Source: CAD feature listing. Evaluate the final solid. Frame: model axes, mm. Face numbers are marked on the shaded views. Round coordinates to 2 decimals unless told otherwise and drop trailing zeros. Order: outer loops, then holes, each group sorted by start corner. A loop starts at its lowest first (then second) coordinate and runs counter-clockwise, first axis right, second up. Notation, with made-up numbers: (-5.75, -28) - (35.25, -28) arc R11 ccw to (35.25, -9) - close; hole circle Ø7 at (52, -7.5). An arc over 180 degrees is marked (long way). Use one line per item in the form item = value. Start each with the question number.
Q1. Pin query (flat end, axial travel): pin 1 Ø1.5 at (x, y) = (7.5, 0) entering from +Z; pin 2 Ø1.6 at (x, y) = (-4, 0) entering from -Z; pin 3 Ø2.5 at (x, y) = (1, 0.5) entering from -Z. Return the tip coordinate at first contact, or that it passes through.
Q2. Ray query, line 1 (Y direction, x = -0.25, z = 2.5); line 2 (Z direction, x = -7.75, y = 0.75); line 3 (X direction, y = -1.25, z = 2.5). Return the intervals inside material, ascending. Write a range as [from, to].
Q3. Draft query along Y for the marked faces 1, 2, 3 and 4. Return one class per face: released by +Y, released by -Y, zero draft, split by the parting line, or undercut.
Q4. Cut plane A-A, the plane z = 0.5. Give the number of separate pieces and of enclosed holes in the cut face, and give its area (3 significant figures).
Q5. Cut plane B-B, the plane x = -6.25. Return the cut outline in (y, z), and give its area (3 significant figures).
Q6. Cut plane D-D, the plane z = 3.05. Return the cut outline in (x, y).
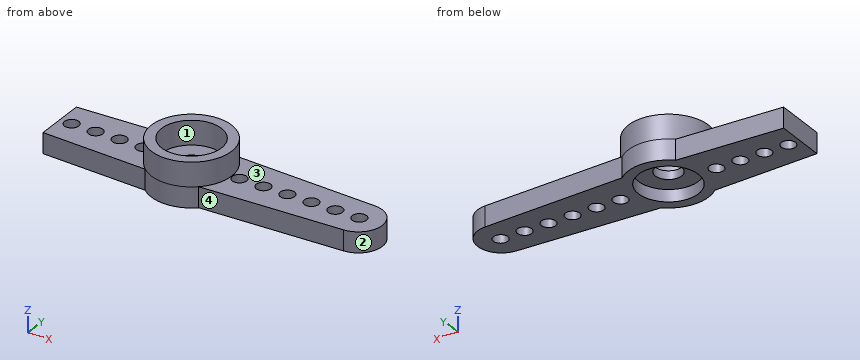
from build123d import *

# Parameters (mm, degrees)
F0_R     = 0.6
F1_DEPTH = 1.7
F2_R     = 3.35
F3_DEPTH = 2
F4_R     = 2.5
F5_DEPTH = 1
F6_R     = 1.1
F7_DEPTH = 2.701
F8_R     = 2.5
F9_DEPTH = 2


with BuildPart() as f1:
    # F0 (on Top) → F1 (new body)
    with BuildSketch(Plane.XY):
        with BuildLine():
            ThreePointArc((2.2299103121, -2.5), (3.057180036, -1.369726333), (3.35, 0))
            ThreePointArc((3.35, 0), (3.057180036, 1.369726333), (2.2299103121, 2.5))
            ThreePointArc((2.2299103121, 2.5), (0, 3.35), (-2.2299103121, 2.5))
            ThreePointArc((-2.2299103121, 2.5), (-3.35, 0), (-2.2299103121, -2.5))
            ThreePointArc((-2.2299103121, -2.5), (0, -3.35), (2.2299103121, -2.5))
        make_face()
        with BuildLine():
            ThreePointArc((2.2299103121, 2.5), (3.057180036, 1.369726333), (3.35, 0))
            ThreePointArc((3.35, 0), (3.057180036, -1.369726333), (2.2299103121, -2.5))
            Line((2.2299103121, -2.5), (14, -2))
            ThreePointArc((14, -2), (15.9168426648, 0), (14, 2))
            Line((14, 2), (2.2299103121, 2.5))
        make_face()
        with Locations((4, 0)):
            Circle(F0_R, mode=Mode.SUBTRACT)
        with Locations((6, 0)):
            Circle(F0_R, mode=Mode.SUBTRACT)
        with Locations((8, 0)):
            Circle(F0_R, mode=Mode.SUBTRACT)
        with Locations((10, 0)):
            Circle(F0_R, mode=Mode.SUBTRACT)
        with Locations((12, 0)):
            Circle(F0_R, mode=Mode.SUBTRACT)
        with Locations((14, 0)):
            Circle(F0_R, mode=Mode.SUBTRACT)
        with BuildLine():
            ThreePointArc((-2.2299103121, -2.5), (-3.35, 0), (-2.2299103121, 2.5))
            Line((-2.2299103121, 2.5), (-11, 2.1274416797))
            Line((-11, 2.1274416797), (-11, -2.1274416797))
            Line((-11, -2.1274416797), (-2.2299103121, -2.5))
        make_face()
        with Locations((-10, 0)):
            Circle(F0_R, mode=Mode.SUBTRACT)
        with Locations((-8, 0)):
            Circle(F0_R, mode=Mode.SUBTRACT)
        with Locations((-6, 0)):
            Circle(F0_R, mode=Mode.SUBTRACT)
        with Locations((-4, 0)):
            Circle(F0_R, mode=Mode.SUBTRACT)
    extrude(amount=F1_DEPTH)

    # F2 (on face) → F3 (join)
    with BuildSketch(Plane.XY.offset(1.7)):
        Circle(F2_R)
    extrude(amount=F3_DEPTH)

    # F4 (on face) → F5 (cut)
    with BuildSketch(Plane(origin=(0, 0, 0), x_dir=(1, 0, 0), z_dir=(0, 0, -1))):
        Circle(F4_R)
    extrude(amount=-F5_DEPTH, mode=Mode.SUBTRACT)

    # F6 (on face) → F7 (cut, through all)
    with BuildSketch(Plane(origin=(0, 0, 1), x_dir=(1, 0, 0), z_dir=(0, 0, -1))):
        Circle(F6_R)
    extrude(amount=-F7_DEPTH, mode=Mode.SUBTRACT)

    # F8 (on face) → F9 (cut)
    with BuildSketch(Plane.XY.offset(3.7)):
        Circle(F8_R)
    extrude(amount=-F9_DEPTH, mode=Mode.SUBTRACT)


solid = f1.part
Completed:
q1.pin_1 = 1.7
q1.pin_2 = 0
q1.pin_3 = 1
q2.line_1 = [-3.34, -2.49], [2.49, 3.34]
q2.line_2 = [0, 1.7]
q2.line_3 = [-3.11, -2.17], [2.17, 3.11]
q3.face_1 = undercut
q3.face_2 = split by the parting line
q3.face_3 = zero draft
q3.face_4 = released by -Y
q4.separate_pieces = 1
q4.enclosed_holes = 11
q4.area = 96.1 mm2
q5.outline = (-2.33, 0) - (-0.55, 0) - (-0.55, 1.7) - (-2.33, 1.7) - close; (0.55, 0) - (2.33, 0) - (2.33, 1.7) - (0.55, 1.7) - close
q5.area = 6.06 mm2
q6.outline = circle Ø6.7 at (0, 0); hole circle Ø5 at (0, 0)
